Source: CAD feature listing. Evaluate the final solid. Frame: model axes, mm. A direction names the side the tool comes from. Coordinates: 2 decimals unless noted, no trailing zeros. Loops run counter-clockwise (first coordinate to the right, second up) from the corner with the lowest first, then second, coordinate; pieces in that order, holes last.
Item 1: Pin query (flat end, axial travel): pin 1 Ø0.8 at (x, y) = (3.5, 4) entering from -Z; pin 2 Ø2.5 at (y, z) = (2, -5.5) entering from -X (3 decimals). Return the tip coordinate at first contact, or that it passes through.
Item 2: Section query B-B, the plane y = 3.05. Return the cut outline in (x, z) (3 decimals), then the cut area to 3 significant figures.
Item 3: Section query C-C, the plane x = 2.25. Return the cut outline in (y, z), then the cut area to 3 significant figures.
Item 4: Line query: probe 1 along X at (y, z) = (3.25, 2) (3 decimals); probe 2 along Z at (x, y) = (2.25, 3.25); probe 3 along Y at (x, z) = (1, 3.5). Output: solid intervals per line, ascending.
Item 5: Section query A-A, the plane z = -1.5. Return the cut outline in (x, y) (3 decimals).
Item 6: Reachability of faces 1 (the flat face through (3, 3, -3.95)), 2 (the cylindrical face through (0.526, 3.083, 1.678)), 3 (the flat face through (4.075, 3, 1)), 4 (the flat face through (0, 6.1, 0)), 5 (the flat face through (-3.075, 3, -5)) from +Z, -Z, +X, -X, +Y, -Y: full face, straight path, thin tool, end or side. Return the list, or none.
Item 7: Section query D-D, the plane z = 5.5. Return the cut outline in (x, y) (3 decimals), then the cut area to 3 significant figures.
Item 8: Pull-direction query (Y, two-part tool) for faces 6 (the flat face through (0, 3, -6.35)), 7 (the cylindrical face through (-0.51, 1.68, 2.41)), 8 (the flat face through (0, 0, 0)); classes: +Y half, -Y half, draft (parallel to the pull), parting line (faces both ways), or undercut.
```python
from build123d import *

# Parameters (mm, degrees)
EXTRUDE_1_DEPTH     = 6.1
SKETCH_2_R          = 2.25
CUT_EXTRUDE_1_DEPTH = 8
SKETCH_3_R          = 0.75
EXTRUDE_2_DEPTH     = 7.5
FILLET_1_R          = 0.75


with BuildPart() as part:
    # Эскиз1 → Бобышка-Вытянуть1 (new body)
    with BuildSketch(Plane(origin=(0, 0, 0), x_dir=(1, 0, 0), z_dir=(0, 1, 0))):
        Polygon((-4.075, 3.95), (-3.075, 3.95), (-3.075, 6.35), (2.425, 6.35), (2.425, 3.95), (4.075, 3.95), (4.075, -6.35), (-4.075, -6.35), align=None)
    extrude(amount=EXTRUDE_1_DEPTH)

    # Эскиз2 → Вырез-Вытянуть1 (cut)
    with BuildSketch(Plane.XY.offset(6.35)):
        with Locations((1.275, 3.05)):
            Circle(SKETCH_2_R)
    extrude(amount=-CUT_EXTRUDE_1_DEPTH, mode=Mode.SUBTRACT)

    # Эскиз3 → Бобышка-Вытянуть2 (add)
    with BuildSketch(Plane.XY.offset(-1.65)):
        with Locations((1.275, 3.05)):
            Circle(SKETCH_3_R)
    extrude(amount=EXTRUDE_2_DEPTH)

    # Скругление1
    fillet_1_edges = [part.edges().sort_by_distance(p)[0] for p in [
        (0.525, 3.05, 5.85),
    ]]
    fillet(fillet_1_edges, radius=FILLET_1_R)


solid = part.part
```
Verdict:
1. pin 1: stops at z = -3.95
1. pin 2: stops at x = -3.075
2. outline: (-4.075, -3.95) - (-3.075, -3.95) - (-3.075, -6.35) - (2.425, -6.35) - (2.425, -3.95) - (4.075, -3.95) - (4.075, 6.35) - (3.525, 6.35) - (3.525, -1.65) - (2.025, -1.65) - (2.025, 5.1) arc R0.75 ccw to (0.525, 5.1) - (0.525, -1.65) - (-0.975, -1.65) - (-0.975, 6.35) - (-4.075, 6.35) - close
2. area: 72.2 mm2
3. outline: (0, -6.35) - (6.1, -6.35) - (6.1, 6.35) - (5.08, 6.35) - (5.08, -1.65) - (1.02, -1.65) - (1.02, 6.35) - (0, 6.35) - close
3. area: 45.0 mm2
4. probe 1: x = -4.075 to -0.966, 0.552 to 1.998, 3.516 to 4.075
4. probe 2: z = -6.35 to -1.65
4. probe 3: y = 0 to 0.82, 2.35 to 3.75, 5.28 to 6.1
5. outline: (-4.075, 0) - (4.075, 0) - (4.075, 6.1) - (-4.075, 6.1) - close; circle Ø1.5 at (1.275, 3.05); hole circle Ø4.5 at (1.275, 3.05)
6. face 1: -Z, +X, +Y, -Y
6. face 2: +Z
6. face 3: +Z, -Z, +X, +Y, -Y
6. face 4: +Z, -Z, +X, -X, +Y
6. face 5: -Z, -X, +Y, -Y
7. outline: (-4.075, 0) - (4.075, 0) - (4.075, 6.1) - (-4.075, 6.1) - close; circle Ø1.269 at (1.275, 3.05); hole circle Ø4.5 at (1.275, 3.05)
7. area: 35.1 mm2
8. face 6: draft
8. face 7: undercut
8. face 8: -Y half
